```python
from build123d import *

# Parameters (mm, degrees)
F1_DEPTH  = 25
F2_R      = 1.55
F3_DEPTH  = 25
F4_R      = 1.5
F5_DEPTH  = 25
F6_R      = 3.313414
F9_DEPTH  = 1.2
F8_R      = 1.5
F10_DEPTH = 1.2
F12_DEPTH = 1.2
F13_R     = 0.5


with BuildPart() as f1:
    # F0 (on Front) → F1 (new body)
    with BuildSketch(Plane.XZ):
        with BuildLine():
            Line((-30, -29.771222), (30, -29.771222))
            Line((30, -29.771222), (30, -19.771222))
            Line((30, -19.771222), (15.039818, -19.771222))
            ThreePointArc((15.039818, -19.771222), (16.48651, -7.699644), (9.500786, 2.251013))
            Line((9.500786, 2.251013), (9.500786, 13.742813))
            Line((9.500786, 13.742813), (3, 13.742813))
            Line((3, 13.742813), (3, 4.886871))
            Line((3, 4.886871), (3, -0.22738))
            ThreePointArc((3, -0.22738), (0, -23.84633), (-3, -0.22738))
            Line((-3, -0.22738), (-3, 4.886871))
            Line((-3, 4.886871), (-3, 13.742813))
            Line((-3, 13.742813), (-9.500786, 13.742813))
            Line((-9.500786, 13.742813), (-9.500786, 2.251013))
            ThreePointArc((-9.500786, 2.251013), (-16.48651, -7.699644), (-15.039818, -19.771222))
            Line((-15.039818, -19.771222), (-30, -19.771222))
            Line((-30, -19.771222), (-30, -29.771222))
        make_face()
    extrude(amount=F1_DEPTH)

    # F2 (on face) → F3 (cut)
    with BuildSketch(Plane.XY.offset(-19.771222)):
        with Locations((-25, -12.5)):
            Circle(F2_R)
        with Locations((25, -12.5)):
            Circle(F2_R)
    extrude(amount=-F3_DEPTH, mode=Mode.SUBTRACT)

    # F4 (on face) → F5 (cut)
    with BuildSketch(Plane.YZ.offset(9.500786)):
        with Locations((-18.75, 7.996913)):
            Circle(F4_R)
        with Locations((-6.25, 7.996913)):
            Circle(F4_R)
    extrude(amount=-F5_DEPTH, mode=Mode.SUBTRACT)

    # F6
    f6_edges = [f1.edges().sort_by_distance(p)[0] for p in [
        (-6.250393, -25, 13.742813),
        (6.250393, -25, 13.742813),
        (-6.250393, 0, 13.742813),
        (6.250393, 0, 13.742813),
        (30, -25, -24.771222),
        (30, 0, -24.771222),
        (-30, 0, -24.771222),
        (-30, -25, -24.771222),
        (15.039818, -12.5, -19.771222),
        (-15.039818, -12.5, -19.771222),
    ]]
    fillet(f6_edges, radius=F6_R)

    # F7 (on face) → F9 (cut)
    with BuildSketch(Plane.YZ.offset(9.500786)):
        Polygon((-20.55, 4.879222), (-16.95, 4.879222), (-15.15, 7.996913), (-16.95, 11.114605), (-20.55, 11.114605), (-22.35, 7.996913), align=None)
        Polygon((-4.45, 11.114605), (-8.05, 11.114605), (-9.85, 7.996913), (-8.05, 4.879222), (-4.45, 4.879222), (-2.65, 7.996913), align=None)
    extrude(amount=-F9_DEPTH, mode=Mode.SUBTRACT)

    # F8 (on face) → F10 (cut)
    with BuildSketch(Plane(origin=(-9.500786, 0, 0), x_dir=(0, -1, 0), z_dir=(-1, 0, 0))):
        Polygon((4.45, 4.879222), (8.05, 4.879222), (9.85, 7.996913), (8.05, 11.114605), (4.45, 11.114605), (2.65, 7.996913), align=None)
        with Locations((6.25, 7.996913)):
            Circle(F8_R, mode=Mode.SUBTRACT)
        Polygon((20.55, 11.114605), (16.95, 11.114605), (15.15, 7.996913), (16.95, 4.879222), (20.55, 4.879222), (22.35, 7.996913), align=None)
        with Locations((18.75, 7.996913)):
            Circle(F8_R, mode=Mode.SUBTRACT)
    extrude(amount=-F10_DEPTH, mode=Mode.SUBTRACT)

    # F11 (on face) → F12 (cut)
    with BuildSketch(Plane.XY.offset(-19.771222)):
        Polygon((26.8, -9.382309), (23.2, -9.382309), (21.4, -12.5), (23.2, -15.617691), (26.8, -15.617691), (28.6, -12.5), align=None)
        Polygon((-23.2, -15.617691), (-21.4, -12.5), (-23.2, -9.382309), (-26.8, -9.382309), (-28.6, -12.5), (-26.8, -15.617691), align=None)
    extrude(amount=-F12_DEPTH, mode=Mode.SUBTRACT)

    # F13
    f13_edges = [f1.edges().sort_by_distance(p)[0] for p in [
        (0, 0, -23.84633),
        (0, -25, -23.84633),
    ]]
    fillet(f13_edges, radius=F13_R)


solid = f1.part
```
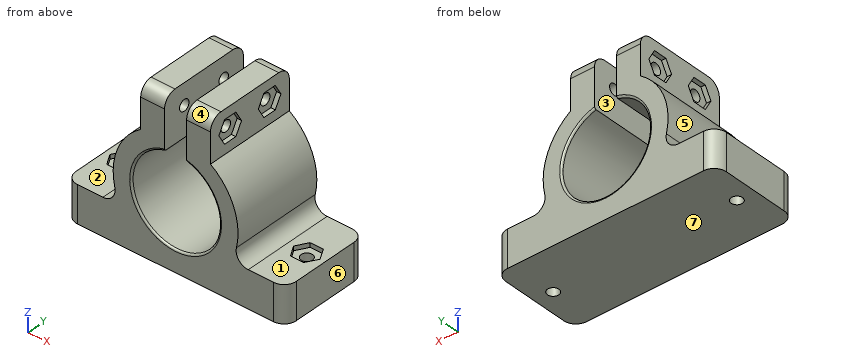
Geometry: final body of the model. Coordinates: model frame, mm. Face numbers are marked on the shaded views. A direction names the side the tool comes from. Give positions to 0.01 mm unless a question says otherwise; leave off trailing zeros. Loops run counter-clockwise (first coordinate to the right, second up) from the corner with the lowest first, then second, coordinate; pieces in that order, holes last. Notation, with made-up numbers: (-20.5, 84.25) - (-16.5, 84.25) arc R10 ccw to (-16.5, 94.25) - close; hole circle Ø8 at (24, 71.5). An arc over 180 degrees is marked (long way). Answer as CSV lines item,"result". Start each with the question number.
(1) Section query C-C (x = 0). Output: boundary loops of the cut face in (y, z), and give its area (3 significant figures).
(2) Section query D-D (x = -19). Output: boundary loops of the cut face in (y, z), and give its area (3 significant figures).
(3) Section query B-B (y = -6.25). Give the number of separate pieces and of enclosed holes in the cut face, and give its area (3 significant figures).
(4) Mould query, pull axis Z, two halves, no side actions, for the marked faces 4, 5, 6 and 7. Classes: +Z half, -Z half, draft (parallel to the pull), parting line (faces both ways), or undercut.
(5) Section query A-A (x = 25). Output: boundary loops of the cut face in (y, z), and give its area (3 significant figures).
(6) Reachability of the marked faces 1, 2 and 3 from +Z, -Z, +X, -X, +Y, -Y: full face, straight path, thin tool, end or side. Return the list, or none.
(7) Ray query, line 1 along X through (y, z) = (-22.75, -11.5) (3 decimals); line 2 along Z through (x, y) = (-6.45, -6.25); line 3 along Z through (x, y) = (5.5, -19.5). Return the intervals inside material, ascending. Write a range as [from, to].
(8) Pin query (flat end, axial travel): P1, Ø10, axis at x = 6, z = -4.5, coming from the -Y side; P2, Ø5, axis at y = -6.25, z = 8, coming from the -X side; P3, Ø11, axis at y = -8, z = 10, coming from the -X side; P4, Ø10, axis at y = -4.5, z = -9, coming from the -X side. Return the tip coordinate at first contact, or that it passes through.
Worked answers:
1,outline,"(-25, -29.77) - (0, -29.77) - (0, -24.35) arc R0.5 ccw to (-0.5, -23.85) - (-24.5, -23.85) arc R0.5 ccw to (-25, -24.35) - close"
1,area,"148 mm^2"
2,outline,"(-25, -29.77) - (0, -29.77) - (0, -19.68) - (-25, -19.68) - close"
2,area,"252 mm^2"
3,separate pieces,"3"
3,enclosed holes,"0"
3,area,"922 mm^2"
4,face 4,"+Z half"
4,face 5,"undercut"
4,face 6,"draft"
4,face 7,"-Z half"
5,outline,"(-25, -29.77) - (-14.05, -29.77) - (-14.05, -20.97) - (-15.62, -20.97) - (-15.62, -19.77) - (-25, -19.77) - close; (-10.95, -29.77) - (0, -29.77) - (0, -19.77) - (-9.38, -19.77) - (-9.38, -20.97) - (-10.95, -20.97) - close"
5,area,"215 mm^2"
6,face 1,"+Z, +X, +Y, -Y"
6,face 2,"+Z, -X, +Y, -Y"
6,face 3,"+Z, +Y, -Y"
7,line 1,"x = [-16.996, -11.995], [11.995, 16.996]"
7,line 2,"z = [-29.77, -21.97], [-1.73, 6.5], [9.5, 13.74]"
7,line 3,"z = [-29.77, -22.51], [-1.18, 6.7], [9.3, 13.74]"
8,P1,"stops at y = -25"
8,P2,"stops at x = -8.3"
8,P3,"stops at x = -9.5"
8,P4,"stops at x = -17"
